Source: CAD feature listing. Evaluate the final solid. Frame: model axes, mm. Face numbers are marked on the shaded views. A direction names the side the tool comes from. Give positions to 0.01 mm unless a question says otherwise; leave off trailing zeros. Order: outer loops, then holes, each group sorted by start corner. A loop starts at its lowest first (then second) coordinate and runs counter-clockwise, first axis right, second up.
from build123d import *

# Parameters (mm, degrees)
F0_R     = 10.16
F2_DEPTH = 19.05
F3_DEPTH = 34.925
F6_DEPTH = 101.6
F7_DEPTH = 101.6


with BuildPart() as f2:
    # F0 (on Top) → F2 (new body)
    with BuildSketch(Plane.XY):
        with BuildLine():
            ThreePointArc((-104.6607, 34.576826), (-80.5307, 10.446826), (-104.6607, -13.683174))
            Line((-104.6607, -13.683174), (-104.6607, -20.42969))
            Line((-104.6607, -20.42969), (-104.6607, -31.54219))
            Line((-104.6607, -31.54219), (-55.142368, -31.54219))
            ThreePointArc((-55.142368, -31.54219), (-51.077865, -31.8695), (-47.118115, -32.842992))
            Line((-47.118115, -32.842992), (-23.892494, -40.576372))
            ThreePointArc((-23.892494, -40.576372), (-19.932744, -41.549864), (-15.868241, -41.877174))
            Line((-15.868241, -41.877174), (15.868241, -41.877174))
            ThreePointArc((15.868241, -41.877174), (19.932744, -41.549864), (23.892494, -40.576372))
            Line((23.892494, -40.576372), (47.118115, -32.842992))
            ThreePointArc((47.118115, -32.842992), (51.077865, -31.8695), (55.142368, -31.54219))
            Line((55.142368, -31.54219), (104.6607, -31.54219))
            Line((104.6607, -31.54219), (104.6607, -20.42969))
            Line((104.6607, -20.42969), (104.6607, -13.683174))
            ThreePointArc((104.6607, -13.683174), (80.5307, 10.446826), (104.6607, 34.576826))
            Line((104.6607, 34.576826), (104.6607, 40.926826))
            Line((104.6607, 40.926826), (104.6607, 52.039326))
            Line((104.6607, 52.039326), (98.910701, 52.039326))
            ThreePointArc((98.910701, 52.039326), (96.758253, 51.663393), (94.860664, 50.580103))
            ThreePointArc((94.860664, 50.580103), (78.004883, 38.780339), (59.468634, 29.849533))
            Line((59.468634, 29.849533), (9.070406, 17.496127))
            ThreePointArc((9.070406, 17.496127), (0, 16.400691), (-9.070406, 17.496127))
            Line((-9.070406, 17.496127), (-59.468634, 29.849533))
            ThreePointArc((-59.468634, 29.849533), (-78.004883, 38.780339), (-94.860664, 50.580103))
            ThreePointArc((-94.860664, 50.580103), (-96.758253, 51.663393), (-98.910701, 52.039326))
            Line((-98.910701, 52.039326), (-104.6607, 52.039326))
            Line((-104.6607, 52.039326), (-104.6607, 40.926826))
            Line((-104.6607, 40.926826), (-104.6607, 34.576826))
        make_face()
        with Locations((0, -19.271174)):
            Circle(F0_R, mode=Mode.SUBTRACT)
    extrude(amount=-F2_DEPTH)

    # F1 (on Top) → F3 (join)
    with BuildSketch(Plane.XY):
        with BuildLine():
            ThreePointArc((-104.6607, -13.683174), (-128.7907, 10.446826), (-104.6607, 34.576826))
            Line((-104.6607, 34.576826), (-104.6607, 52.039326))
            Line((-104.6607, 52.039326), (-109.834866, 52.039326))
            ThreePointArc((-109.834866, 52.039326), (-113.950863, 51.353842), (-117.622536, 49.371385))
            Line((-117.622536, 49.371385), (-134.142671, 36.547162))
            ThreePointArc((-134.142671, 36.547162), (-137.797157, 32.025737), (-139.053922, 26.349551))
            Line((-139.053922, 26.349551), (-138.634187, -5.846879))
            ThreePointArc((-138.634187, -5.846879), (-137.371916, -11.203376), (-133.962188, -15.522999))
            Line((-133.962188, -15.522999), (-117.690247, -28.794484))
            ThreePointArc((-117.690247, -28.794484), (-113.92365, -30.916909), (-109.663324, -31.652812))
            Line((-109.663324, -31.652812), (-104.6607, -31.652812))
            Line((-104.6607, -31.652812), (-104.6607, -13.683174))
        make_face()
        with BuildLine():
            ThreePointArc((117.622536, 49.371385), (113.950863, 51.353842), (109.834866, 52.039326))
            Line((109.834866, 52.039326), (104.6607, 52.039326))
            Line((104.6607, 52.039326), (104.6607, 34.576826))
            ThreePointArc((104.6607, 34.576826), (128.7907, 10.446826), (104.6607, -13.683174))
            Line((104.6607, -13.683174), (104.6607, -31.652812))
            Line((104.6607, -31.652812), (109.663324, -31.652812))
            ThreePointArc((109.663324, -31.652812), (113.92365, -30.916909), (117.690247, -28.794484))
            Line((117.690247, -28.794484), (133.962188, -15.522999))
            ThreePointArc((133.962188, -15.522999), (137.371916, -11.203376), (138.634187, -5.846879))
            Line((138.634187, -5.846879), (139.053922, 26.349551))
            ThreePointArc((139.053922, 26.349551), (137.797157, 32.025737), (134.142671, 36.547162))
            Line((134.142671, 36.547162), (117.622536, 49.371385))
        make_face()
    extrude(amount=-F3_DEPTH)

    # F5 (on offset) → F6 (cut)
    with BuildSketch(Plane.XZ.offset(31.5468)):
        Polygon((-104.723774, -19.364603), (-138.805479, -34.856286), (-138.805479, -39.619088), (-104.723774, -39.619088), (-104.723774, -38.741853), (-97.308874, -38.741853), (-97.308874, -19.364603), align=None)
        Polygon((104.723774, -19.364603), (97.308874, -19.364603), (97.308874, -38.741853), (104.723774, -38.741853), (104.723774, -39.619088), (138.805479, -39.619088), (138.805479, -34.856286), align=None)
    extrude(amount=-F6_DEPTH, mode=Mode.SUBTRACT)

    # F5 (on offset) → F7 (cut)
    with BuildSketch(Plane.XZ.offset(31.5468)):
        Polygon((-104.723774, -19.364603), (-138.805479, -34.856286), (-138.805479, -39.619088), (-104.723774, -39.619088), (-104.723774, -38.741853), (-97.308874, -38.741853), (-97.308874, -19.364603), align=None)
        Polygon((104.723774, -19.364603), (97.308874, -19.364603), (97.308874, -38.741853), (104.723774, -38.741853), (104.723774, -39.619088), (138.805479, -39.619088), (138.805479, -34.856286), align=None)
    extrude(amount=-F7_DEPTH, mode=Mode.SUBTRACT)


solid = f2.part
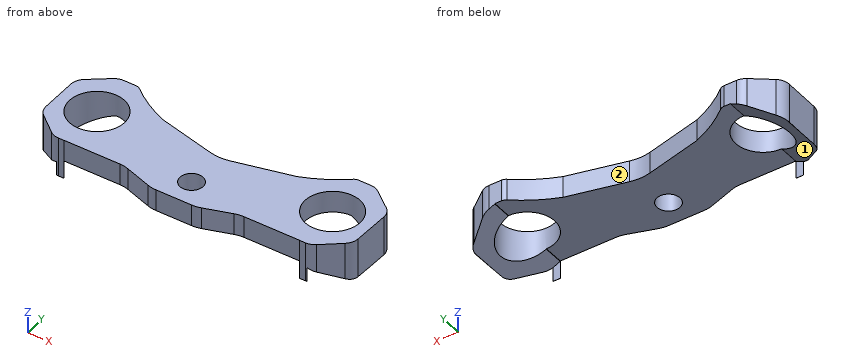
1) First-contact query: pin 1 Ø6 at (y, z) = (40.5, -13.5) entering from +X; pin 2 Ø23.5 at (x, y) = (0, -19.27) entering from -Z; pin 3 Ø5 at (x, z) = (-88.5, -21) entering from -Y. Flat tips, straight axial feed; report the tip coordinate or a pass-through.
Checks:
pin 1: stops at x = 132.92
pin 2: stops at z = -19.05
pin 3: stops at y = -31.54
2) Ray query, L1, parallel to Y at x = 106, z = -13.5; L2, parallel to X at y = 11.5, z = -5; L3, parallel to Y at x = 0, z = -14.25. Return the intervals inside material, ascending.
Checks:
L1: y = -31.65 to -13.65, 34.54 to 52.04
L2: x = -138.86 to -128.77, -80.55 to 80.55, 128.77 to 138.86
L3: y = -41.88 to -29.43, -9.11 to 16.4
3) Section query D-D on z = -2.5. State how many separate pieces and enclosed holes the cut face has, and give its area (3 significant figures).
Checks:
separate pieces: 1
enclosed holes: 3
area: 14,500 mm2
4) Reachability of the marked faces 1 and 2 from +Z, -Z, +X, -X, +Y, -Y: full face, straight path, thin tool, end or side. Return the list, or none.
Checks:
face 1: -Z, +Y
face 2: +Z, -Z, +Y
5) Section query A-A on x = 0. Output: boundary loops of the cut face in (y, z), and give its area (3 significant figures).
Checks:
outline: (-41.88, -19.05) - (-29.43, -19.05) - (-29.43, 0) - (-41.88, 0) - close; (-9.11, -19.05) - (16.4, -19.05) - (16.4, 0) - (-9.11, 0) - close
area: 723 mm2
6) Section query B-B on y = -24. Output: boundary loops of the cut face in (x, z).
Checks:
outline: (-123.57, -27.93) - (-104.72, -19.36) - (-104.66, -19.36) - (-104.66, -19.05) - (-8.99, -19.05) - (-8.99, 0) - (-123.57, 0) - close; (8.99, -19.05) - (104.66, -19.05) - (104.66, -19.36) - (104.72, -19.36) - (123.57, -27.93) - (123.57, 0) - (8.99, 0) - close
7) Section query C-C on x = 88. Output: boundary loops of the cut face in (y, z), and give its area (3 significant figures).
Checks:
outline: (-31.54, -19.05) - (-7.01, -19.05) - (-7.01, 0) - (-31.54, 0) - close; (27.9, -19.05) - (45.28, -19.05) - (45.28, 0) - (27.9, 0) - close
area: 798 mm2
